Verification items for the finished model (mm, model axes). Face numbers are marked on the shaded views. Give positions to 0.01 mm unless a question says otherwise; leave off trailing zeros. Write each loop counter-clockwise with the first axis right and the second up, starting at its lowest first coordinate (ties: lowest second). Pieces come first, ordered by that corner, then holes. Notation, with made-up numbers: (6, 7) -> (49, 7) arc R18 cw to (49, 42) -> close; hole circle Ø6 at (-3, -0.75). An arc over 180 degrees is marked (long way). Use CSV: the item, a comma, the result in double quotes. Start each with the question number.
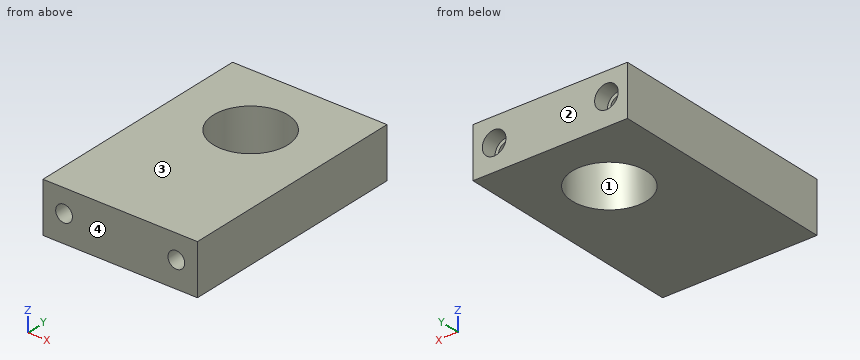
Autodesk Inventor part; units mm, degrees
ref_plane "YZ Plane" through (0, 0, 0) normal (1, 0, 0) x (0, 1, 0)
ref_plane "XZ Plane" through (0, 0, 0) normal (0, 1, 0) x (-1, 0, 0)
ref_plane "XY Plane" through (0, 0, 0) normal (0, 0, 1) x (1, 0, 0)
sketch "Sketch1" plane through (0, 0, 0) normal (0, 0, 1) x (1, 0, 0)
  circle A0 centre (22.919, 29.5195) radius 18.75
  line L0 (-15.9938, 66.3532) -> (61.8383, 66.3532)
  line L1 (61.8383, 66.3532) -> (61.8383, -51.7605)
  line L2 (61.8383, -51.7605) -> (-15.9938, -51.7605)
  line L3 (-15.9938, -51.7605) -> (-15.9938, 66.3532)
  point P0 (0, 0)
  dimension "d0" = 37.5
  dimension "d1" = 77.8321
  dimension "d2" = 118.1137
  dimension "d3" = 38.9128
  dimension "d4" = 81.28
extrude "Extrusion1" add sketch "Sketch1" along normal blind 25.4
sketch "Sketch2" plane through (-15.9938, 66.3532, 0) normal (0, 1, 0) x (1, 0, 0)
  point P0 (15.9938, 0)
  point P1 (10.6081, -13.72)
hole "Hole1" at (-5.3858, 66.3532, 13.72) direction (0, -1, 0) diameter 8.4328 end through all counterbore diameter 11.9062 counterbore depth 7.9502
sketch "Sketch3" plane through (-15.9938, 66.3532, 0) normal (0, 1, 0) x (1, 0, 0)
  point P0 (15.9938, 0)
  point P1 (67.1861, -13.2652)
hole "Hole2" at (51.1923, 66.3532, 13.2652) direction (0, -1, 0) diameter 8.4328 end through all counterbore diameter 11.9062 counterbore depth 7.9502
properties part number "Wrist Support"
(1) Section check B-B on y = 18. Record the cut outline in (x, z), then the cut area to 3 significant figures.
(2) Section check A-A on z = 13.72. Record the cut outline in (x, y).
(3) Go/stop test with flat-tipped pins: pin 1 (13 mm diameter, centred on x = 50, z = 14.5, fed in from +Y); pin 2 (7 mm diameter, centred on x = -5.39, z = 13.72, fed in from +Y). Record where each tip stops, or that it passes through.
(4) Section check C-C on x = 22. Record the cut outline in (y, z), then the cut area to 3 significant figures.
(5) Draft check along Y on the marked faces 1, 2, 3 and 4. Enter one of: released by +Y, released by -Y, zero draft, split by the parting line, or undercut.
(6) Section check D-D on y = -22. Record the cut outline in (x, z), then the cut area to 3 significant figures.
(7) Thickness scan on line 1 (X direction, y = -43.5, z = 13.75); line 2 (X direction, y = -8, z = 15); line 3 (Y direction, x = 23.5, z = 12.25). Record the ranges inside material, lowest first. Write a range as from..to.
Data:
1,outline,"(-15.99, 0) -> (8.12, 0) -> (8.12, 25.4) -> (-15.99, 25.4) -> close; (37.71, 0) -> (61.84, 0) -> (61.84, 25.4) -> (37.71, 25.4) -> close; hole circle Ø8.43 at (-5.39, 13.72); hole circle Ø8.43 at (51.19, 13.27)"
1,area,"1,110 mm2"
2,outline,"(-15.99, -51.76) -> (-9.6, -51.76) -> (-9.6, 58.4) -> (-11.34, 58.4) -> (-11.34, 66.35) -> (-15.99, 66.35) -> close; (-1.17, -51.76) -> (47, -51.76) -> (47, 58.4) -> (45.26, 58.4) -> (45.26, 66.35) -> (0.57, 66.35) -> (0.57, 58.4) -> (-1.17, 58.4) -> close; (55.38, -51.76) -> (61.84, -51.76) -> (61.84, 66.35) -> (57.13, 66.35) -> (57.13, 58.4) -> (55.38, 58.4) -> close; hole circle Ø37.5 at (22.92, 29.52)"
3,pin 1,"stops at y = 66.35"
3,pin 2,"passes through"
4,outline,"(-51.76, 0) -> (10.79, 0) -> (10.79, 25.4) -> (-51.76, 25.4) -> close; (48.25, 0) -> (66.35, 0) -> (66.35, 25.4) -> (48.25, 25.4) -> close"
4,area,"2,050 mm2"
5,face 1,"undercut"
5,face 2,"released by +Y"
5,face 3,"zero draft"
5,face 4,"released by -Y"
6,outline,"(-15.99, 0) -> (61.84, 0) -> (61.84, 25.4) -> (-15.99, 25.4) -> close; hole circle Ø8.43 at (-5.39, 13.72); hole circle Ø8.43 at (51.19, 13.27)"
6,area,"1,870 mm2"
7,line 1,"x = -15.99..-9.6, -1.17..47, 55.38..61.84"
7,line 2,"x = -15.99..-9.4, -1.37..47.35, 55.04..61.84"
7,line 3,"y = -51.76..10.78, 48.26..66.35"
